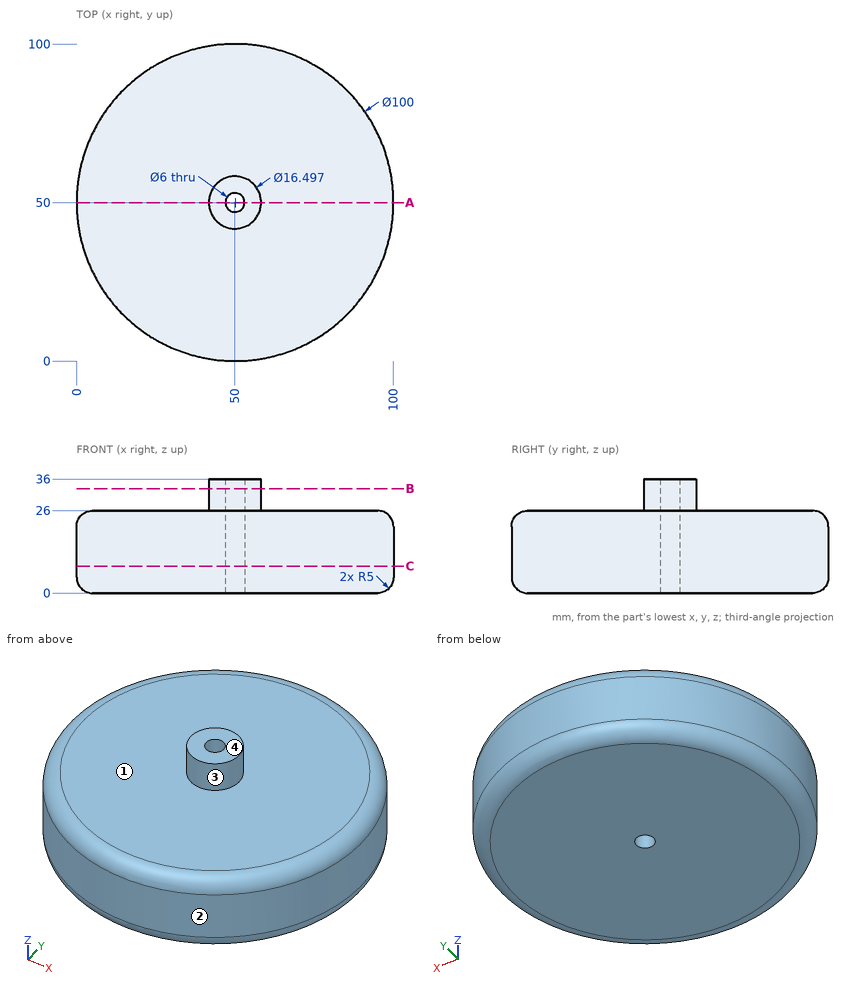
Geometry: see drawing. Coordinates: mm, zero at the bounding-box minimum. A direction names the side the tool comes from. Round coordinates to 2 decimals unless told otherwise and drop trailing zeros. Loops run counter-clockwise (first coordinate to the right, second up) from the corner with the lowest first, then second, coordinate; pieces in that order, holes last. Notation, with made-up numbers: (55.5, 75) -> (111.5, 75) arc R28 cw to (111.5, 106) -> close; hole circle Ø8 at (-9.5, 22.25). An arc over 180 degrees is marked (long way). Use one line per item in the form item = value. Start each with the question number.
Item 1: Mould query, pull axis X, two halves, no side actions, for the marked faces 1 and 2. Classes: pulls with the +X half, pulls with the -X half, needs draft (parallel to the pull), parting line crosses it, or undercut.
Item 2: Section query A-A on y = 50. Return the cut outline in (x, z), then the cut area to 3 significant figures.
Item 3: Section query B-B on z = 33. Return the cut outline in (x, y).
Item 4: Set-up query: the marked faces 3 and 4. Return all of +Z, -Z, +X, -X, +Y, -Y with unobstructed straight access to the full face (end or side cutting, diameter ignored); none if empty.
Item 5: Contact query for flat-ended pins moving along their axis: pin 1 Ø12 at (y, z) = (66.5, 26.5) entering from +X; pin 2 Ø8 at (x, z) = (75, 17.5) entering from +Y; pin 3 Ø4 at (y, z) = (61.5, 5) entering from -X. Output: stop coordinate, or through.
Item 6: Material intervals for L1, parallel to Y at x = 50, z = 17.5; L2, parallel to Z at x = 83.5, y = 58; L3, parallel to X at y = 49, z = 23.5, sorted ascending. Write a range as from..to.
Item 7: Section query C-C on z = 8.5. Return the cut outline in (x, y), then the cut area to 3 significant figures.
Ans:
q1.face_1 = needs draft
q1.face_2 = parting line crosses it
q2.outline = (0, 5) arc R5 ccw to (5, 0) -> (47, 0) -> (47, 36) -> (41.75, 36) -> (41.75, 26) -> (5, 26) arc R5 ccw to (0, 21) -> close; (53, 0) -> (95, 0) arc R5 ccw to (100, 5) -> (100, 21) arc R5 ccw to (95, 26) -> (58.25, 26) -> (58.25, 36) -> (53, 36) -> close
q2.area = 2,530 mm^2
q3.outline = circle Ø16.5 at (50, 50); hole circle Ø6 at (50, 50)
q4.face_3 = +Z
q4.face_4 = +Z, +X, -X, +Y, -Y
q5.pin_1 = 98.31
q5.pin_2 = 95.38
q5.pin_3 = 0.91
q6.L1 = 0..47, 53..100
q6.L2 = 0..26
q6.L3 = 0.68..47.17, 52.83..99.32
q7.outline = circle Ø100 at (50, 50); hole circle Ø6 at (50, 50)
q7.area = 7,830 mm^2
